Read the model definition and answer for the solid it produces. Units are mm, in the model's axes. A direction names the side the tool comes from. Give positions to 0.01 mm unless a question says otherwise; leave off trailing zeros. Write each loop counter-clockwise with the first axis right and the second up, starting at its lowest first coordinate (ties: lowest second). Pieces come first, ordered by that corner, then holes. Notation, with made-up numbers: M 70,67 L 78,67 A20 ccw 78,104 Z; hole C 50,-27.75 d9. An arc over 180 degrees is marked long. Answer as CSV lines item,"result". Start each with the question number.
```python
from build123d import *

# Parameters (mm, degrees)
F0_W         = 1.7
F0_H         = 47.6
F1_DEPTH     = 35.2
F2_DEPTH     = 1.5
F3_T4_DEPTH  = 42.5422275002
F3_T9_DEPTH  = 56.4422275002
F3_T14_DEPTH = 42.5422275002
F5_DEPTH     = 0.8


# Not quite as in the source:
# - a fillet or chamfer that OpenCascade refuses, or shapes differently, is made with other operations: its cross-section is extruded or revolved along the edge and cut away or added
# - ends of sketch curves that miss each other by under 0.0002 mm in the source are joined


with BuildPart() as f1:
    # F0 (on Top) → F1 (new body)
    with BuildSketch(Plane.XY):
        Polygon((21.457163617, -2.1686828911), (21.457163617, -52.9686828911), (23.757163617, -52.9686828911), (23.757163617, -51.3686828911), (23.757163617, -3.7686828911), (23.757163617, -2.1686828911), align=None)
        with Locations((24.607163617, -27.5686828911)):
            Rectangle(F0_W, F0_H)
    extrude(amount=F1_DEPTH)

    # F0 (on Top) → F2 (cut)
    with BuildSketch(Plane.XY):
        with Locations((24.607163617, -27.5686828911)):
            Rectangle(F0_W, F0_H)
    extrude(amount=F2_DEPTH, mode=Mode.SUBTRACT)

    # F3: chamfer of 0.3 x 1.7013845459 on 3 edges, made by hand


with BuildPart() as f3_tool2:
    # F3_s3 → F3_t4 (new body)
    with BuildSketch(Plane.XY.offset(-2.9211137501)):
        Polygon((25.457163617, -51.0686828911), (23.7557790711, -51.3686828911), (25.457163617, -51.3686828911), align=None)
    extrude(amount=F3_T4_DEPTH)

    split(bisect_by=Plane.YZ.offset(23.757163617), keep=Keep.TOP)


with BuildPart() as f1_1:
    add(f1.part)

    # F3_t1: cut F3_tool2
    add(f3_tool2.part, mode=Mode.SUBTRACT)


with BuildPart() as f3_tool7:
    # F3_s8 → F3_t9 (new body)
    with BuildSketch(Plane.XZ.offset(55.7897966412)):
        Polygon((23.7557790711, 1.5), (25.457163617, 1.8), (25.457163617, 1.5), align=None)
    extrude(amount=-F3_T9_DEPTH)

    split(bisect_by=Plane.YZ.offset(23.757163617), keep=Keep.TOP)


with BuildPart() as f1_2:
    add(f1_1.part)

    # F3_t6: cut F3_tool7
    add(f3_tool7.part, mode=Mode.SUBTRACT)


with BuildPart() as f3_tool12:
    # F3_s13 → F3_t14 (new body)
    with BuildSketch(Plane.XY.offset(-2.9211137501)):
        Polygon((23.7557790711, -3.7686828911), (25.457163617, -4.0686828911), (25.457163617, -3.7686828911), align=None)
    extrude(amount=F3_T14_DEPTH)

    split(bisect_by=Plane.YZ.offset(23.757163617), keep=Keep.TOP)


with BuildPart() as f1_3:
    add(f1_2.part)

    # F3_t11: cut F3_tool12
    add(f3_tool12.part, mode=Mode.SUBTRACT)

    # F4 (on face) → F5 (cut)
    with BuildSketch(Plane.YZ.offset(25.457163617)):
        Polygon((-24.0221414911, 13.6708992), (-24.0221414911, 12.9445354), (-24.0221414911, 12.2181716), (-21.7966950911, 12.2181716), (-19.5712486911, 12.2181716), (-19.5712486911, 12.9445354), (-19.5712486911, 13.6708992), (-21.7966950911, 13.6708992), align=None)
        Polygon((-24.0221414911, 9.9618134), (-24.0221414911, 9.2354496), (-24.0221414911, 8.5090858), (-21.7966950911, 8.5090858), (-19.5712486911, 8.5090858), (-19.5712486911, 9.2354496), (-19.5712486911, 9.9618134), (-21.7966950911, 9.9618134), align=None)
        Polygon((-18.0566974911, 6.280566), (-18.0566974911, 5.5376414), (-18.0566974911, 4.7947676), (-16.9207840911, 4.807493), (-15.5376016911, 4.8880872), (-14.2955670911, 5.6452866), (-13.8898274911, 6.2280134), (-13.6151518911, 7.2483822), (-14.0528446911, 8.8343074), (-15.3985112911, 9.8445416), (-15.6921352911, 9.9462178), (-16.8744290911, 9.9559968), (-18.0566974911, 9.9658012), (-18.0566974911, 9.2389548), (-18.0566974911, 8.512083), (-16.9818456911, 8.5028628), (-15.9070192911, 8.4936172), (-15.7007458911, 8.3920426), (-15.0843894911, 7.5677364), (-15.2217272911, 6.8451064), (-15.7842102911, 6.3483586), (-17.0050104911, 6.2828266), align=None)
        Polygon((-12.8639722911, 8.4833048), (-11.0016950911, 6.6416524), (-9.1394178911, 4.8), (-8.1040376911, 4.8), (-7.0686828911, 4.8), (-9.2939768911, 7.0254464), (-11.5192454911, 9.2508928), (-9.3094200911, 11.460896), (-7.0995692911, 13.6708992), (-8.1350510911, 13.6708992), (-9.1705328911, 13.6708992), (-11.0172398911, 11.823989), (-12.8639722911, 9.9770788), (-12.8639722911, 9.2301918), align=None)
    extrude(amount=-F5_DEPTH, mode=Mode.SUBTRACT)


solid = f1_3.part
```
1. Find section A-A on z = 15. Determine the outline of the cut face in (x, y), then the cut area to 3 significant figures.
2. Determine the mould class of faces 1 (the face through (24.595, -3.917, 18.114)), 2 (the face through (23, -52.969, 17)), 3 (the face through (25.06, -11.03, 6.67)), 4 (the face through (25.457, -28, 18)) for opening direction Y: +Y half, -Y half, draft (parallel to the pull), parting line (faces both ways), or undercut.
3. Find section C-C on y = -25. Determine the outline of the cut face in (x, z).
4. Find section B-B on y = -10. Determine the outline of the cut face in (x, z).
5. Find the intervals of material crossed by line 1 (Z direction, x = 24.75, y = -22.5); line 2 (Y direction, x = 24.8, z = 6.5); line 3 (Y direction, x = 24.1, z = 15), in increasing order. Write a range as [from, to].
6. For faces 5 (the face through (24.657, -22, 13)), 6 (the face through (23, -27, 0)), 7 (the face through (23.757, -28, 1)), determine the directions among +Z, -Z, +X, -X, +Y, -Y from which every point of the face is accessible in a straight line to the end or side of a thin tool.
7. Given pin 1 (0.6 mm diameter, centred on x = 25, z = 6, fed in from +Y); pin 2 (0.6 mm diameter, centred on x = 25, y = -21.5, fed in from -Z), each flat-ended and moving along its own axis, determine where each tip first touches the part or whether it passes through.
Computed:
1,outline,"M 21.46,-52.97 L 23.76,-52.97 L 23.76,-51.37 L 25.46,-51.07 L 25.46,-4.07 L 23.76,-3.77 L 23.76,-2.17 L 21.46,-2.17 Z"
1,area,"197 mm^2"
2,face 1,"+Y half"
2,face 2,"-Y half"
2,face 3,"undercut"
2,face 4,"draft"
3,outline,"M 21.46,0 L 23.76,0 L 23.76,1.5 L 25.46,1.8 L 25.46,35.2 L 21.46,35.2 Z"
4,outline,"M 21.46,0 L 23.76,0 L 23.76,1.5 L 25.46,1.8 L 25.46,5.65 L 24.66,5.65 L 24.66,7.73 L 25.46,7.73 L 25.46,10.77 L 24.66,10.77 L 24.66,12.84 L 25.46,12.84 L 25.46,35.2 L 21.46,35.2 Z"
5,line 1,"z = [1.68, 8.51], [9.96, 12.22], [13.67, 35.2]"
5,line 2,"y = [-51.18, -15.61], [-13.82, -10.86], [-8.77, -3.95]"
5,line 3,"y = [-51.31, -3.83]"
6,face 5,"+X"
6,face 6,"-Z, +X, -X, +Y, -Y"
6,face 7,"-Z, +X"
7,pin 1,"stops at y = -3.94"
7,pin 2,"stops at z = 1.67"
